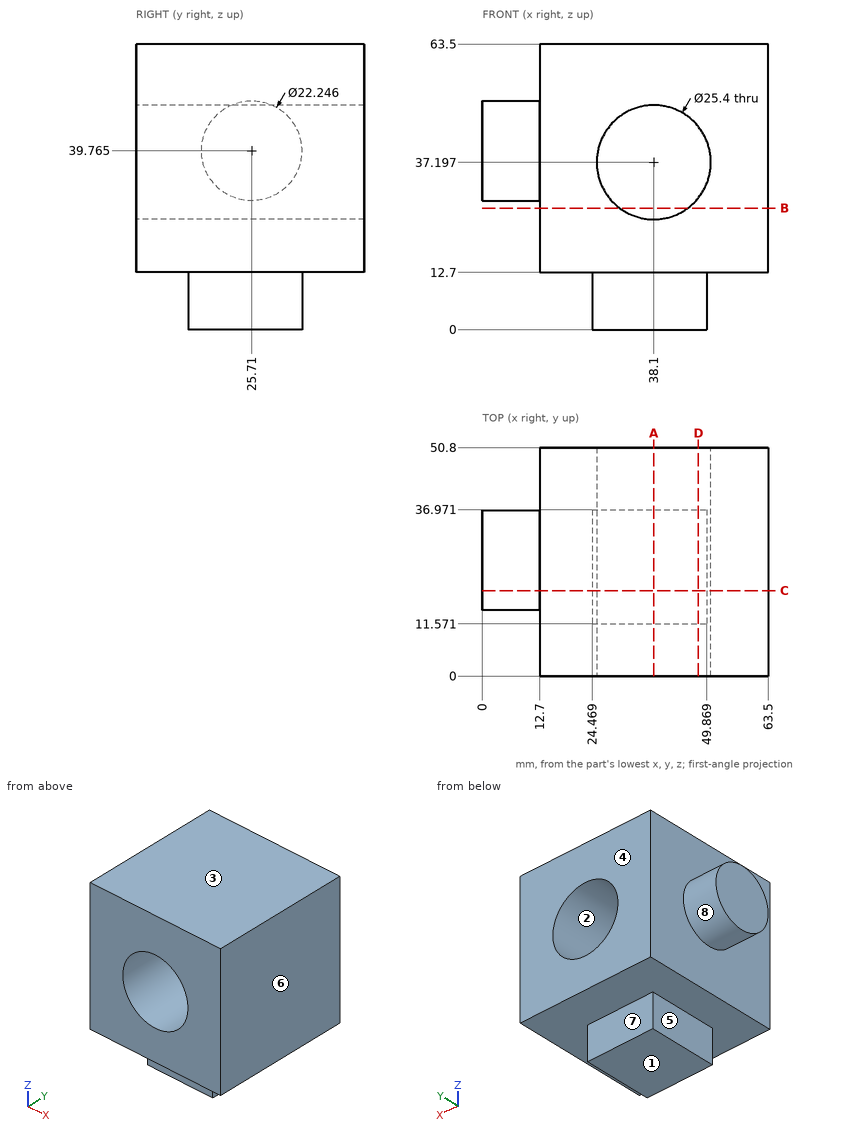
Could you check a few things on this drawing? It's one solid part, dimensions in mm from its lowest x, y, z. A direction names the side the tool comes from. Give positions to 0.01 mm unless a question says otherwise; leave off trailing zeros. Order: outer loops, then holes, each group sorted by start corner. A loop starts at its lowest first (then second) coordinate and runs counter-clockwise, first axis right, second up. Notation, with made-up numbers: (64, -5.5) -> (92, -5.5) arc R25 cw to (92, 7.5) -> close; hole circle Ø10 at (1.25, 63). An arc over 180 degrees is marked (long way). Use CSV: the item, a comma, the result in double quotes. Start each with the question number.
Item 1: I'm going to push flat-ended pins straight in: P1, Ø8, axis at y = 10.5, z = 9, coming from the -X side; P2, Ø4, axis at x = 12.5, z = 10, coming from the -Y side; P3, Ø6.5, axis at x = 36, z = 7, coming from the +Y side; P4, Ø10, axis at x = 41, z = 7, coming from the -Y side. Where does each tip first touch, or does it pass through?
Item 2: If I drill on probe 1 along Z at (x, y) = (38.1, 35.5); probe 2 along Z at (x, y) = (38.1, 37.5); probe 3 along Z at (x, y) = (18.5, 18), over which ranges is the centre line in solid material (lowest first)? Write a range as [from, to].
Item 3: Suppose I cut it at C-C (y = 19). List the corners of the cut face in (x, z) for me (1 decimal).
Item 4: Suppose I cut it at B-B (z = 27). List the corners of the cut face in (x, y) for me.
Item 5: Suppose I cut it at D-D (x = 48). List the corners of the cut face in (y, z) for me.
Item 6: On a 3-axis mill with a long thin cutter (end or side, diameter ignored), from which of +Z, -Z, +X, -X, +Y, -Y can I reach the whole of each face in a straight line? I mean the marked faces 5, 6, 7 and 8. Say none if no direction works.
Item 7: Thinking about a two-plate mould opening in Z: for the marked faces 1, 2, 3 and 4, which applies, pulls with the +Z half, pulls with the -Z half, needs draft (parallel to the pull), parting line crosses it, or undercut?
Item 8: Suppose I cut it at A-A (x = 38.1). List the corners of the cut face in (y, z) for me, and give its area (3 significant figures).
Answer block:
1,P1,"stops at x = 12.7"
1,P2,"passes through"
1,P3,"stops at y = 36.97"
1,P4,"stops at y = 11.57"
2,probe 1,"z = [0, 24.5], [49.9, 63.5]"
2,probe 2,"z = [12.7, 24.5], [49.9, 63.5]"
2,probe 3,"z = [12.7, 63.5]"
3,outline,"(0, 30.9) -> (12.7, 30.9) -> (12.7, 12.7) -> (24.5, 12.7) -> (24.5, 0) -> (49.9, 0) -> (49.9, 12.7) -> (63.5, 12.7) -> (63.5, 63.5) -> (12.7, 63.5) -> (12.7, 48.6) -> (0, 48.6) -> close; hole circle Ø25.4 at (38.1, 37.2)"
4,outline,"(12.7, 0) -> (30.53, 0) -> (30.53, 50.8) -> (12.7, 50.8) -> close; (45.67, 0) -> (63.5, 0) -> (63.5, 50.8) -> (45.67, 50.8) -> close"
5,outline,"(0, 12.7) -> (11.57, 12.7) -> (11.57, 0) -> (36.97, 0) -> (36.97, 12.7) -> (50.8, 12.7) -> (50.8, 29.24) -> (0, 29.24) -> close; (0, 45.15) -> (50.8, 45.15) -> (50.8, 63.5) -> (0, 63.5) -> close"
6,face 5,"-Z, -X, +Y, -Y"
6,face 6,"+Z, -Z, +X, +Y, -Y"
6,face 7,"-Z, +X, -X, +Y"
6,face 8,"-X"
7,face 1,"pulls with the -Z half"
7,face 2,"undercut"
7,face 3,"pulls with the +Z half"
7,face 4,"needs draft"
8,outline,"(0, 12.7) -> (11.57, 12.7) -> (11.57, 0) -> (36.97, 0) -> (36.97, 12.7) -> (50.8, 12.7) -> (50.8, 24.5) -> (0, 24.5) -> close; (0, 49.9) -> (50.8, 49.9) -> (50.8, 63.5) -> (0, 63.5) -> close"
8,area,"1,610 mm^2"
